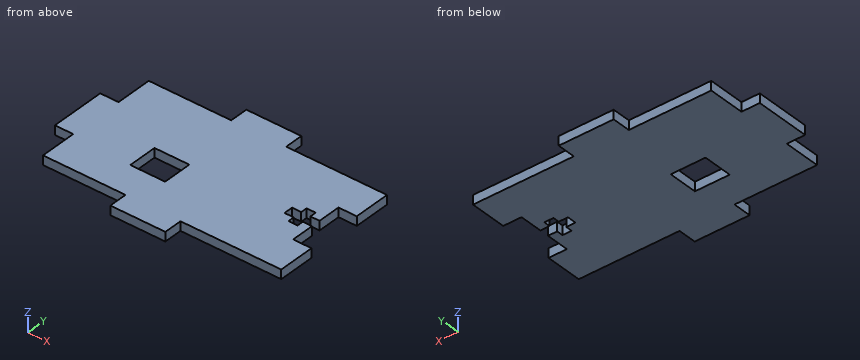
```python
from build123d import *

# Parameters (mm, degrees)
SKETCH1_W           = 82.55
SKETCH1_H           = 44.45
BOSS_EXTRUDE1_DEPTH = 3.175
SKETCH2_W           = 6.35
SKETCH2_H           = 19.05
BOSS_EXTRUDE2_DEPTH = 3.175
SKETCH5_W           = 19.05
SKETCH5_H           = 6.35
BOSS_EXTRUDE3_DEPTH = 3.175
SKETCH3_W           = 6.35
SKETCH3_H           = 19.05
CUT_EXTRUDE1_DEPTH  = 3.175
SKETCH6_W           = 12.065
SKETCH6_H           = 10.16
CUT_EXTRUDE2_DEPTH  = 97.980529618
CUT_EXTRUDE3_DEPTH  = 97.980529618


with BuildPart() as part:
    # Sketch1 → Boss-Extrude1 (new body)
    with BuildSketch(Plane.XY):
        with Locations((41.275, 22.225)):
            Rectangle(SKETCH1_W, SKETCH1_H)
    extrude(amount=BOSS_EXTRUDE1_DEPTH)

    # Sketch2 → Boss-Extrude2 (add)
    with BuildSketch(Plane.XY.offset(3.175)):
        with Locations((-3.175, 22.225)):
            Rectangle(SKETCH2_W, SKETCH2_H)
    extrude(amount=-BOSS_EXTRUDE2_DEPTH)

    # Sketch5 → Boss-Extrude3 (add)
    with BuildSketch(Plane.XY.offset(3.175)):
        with Locations((38.1, 47.625)):
            Rectangle(SKETCH5_W, SKETCH5_H)
        with Locations((38.1, -3.175)):
            Rectangle(SKETCH5_W, SKETCH5_H)
    extrude(amount=-BOSS_EXTRUDE3_DEPTH)

    # Sketch3 → Cut-Extrude1 (cut)
    with BuildSketch(Plane.XY.offset(3.175)):
        with Locations((79.375, 22.225)):
            Rectangle(SKETCH3_W, SKETCH3_H)
    extrude(amount=-CUT_EXTRUDE1_DEPTH, mode=Mode.SUBTRACT)

    # Sketch6 → Cut-Extrude2 (cut, through all)
    with BuildSketch(Plane.XY.offset(3.175)):
        with Locations((26.8605, 16.51)):
            Rectangle(SKETCH6_W, SKETCH6_H)
    extrude(amount=-CUT_EXTRUDE2_DEPTH, mode=Mode.SUBTRACT)

    # Sketch7 → Cut-Extrude3 (cut, through all)
    with BuildSketch(Plane.XY.offset(3.175)):
        Polygon((69.85, 26.035), (73.025, 26.035), (73.025, 23.8125), (76.2, 23.8125), (76.2, 20.6375), (73.025, 20.6375), (73.025, 18.415), (69.85, 18.415), (69.85, 20.6375), (66.675, 20.6375), (66.675, 23.8125), (69.85, 23.8125), align=None)
    extrude(amount=-CUT_EXTRUDE3_DEPTH, mode=Mode.SUBTRACT)


solid = part.part
```
Check sheet for the modelled part. Datum: model origin and axes. Units: mm. Round coordinates to 2 decimals unless told otherwise and drop trailing zeros. Order: outer loops, then holes, each group sorted by start corner. A loop starts at its lowest first (then second) coordinate and runs counter-clockwise, first axis right, second up. Notation, with made-up numbers: M 78.5,-6 L 125.5,-6 A14 cw 125.5,11 Z; hole C 22.25,-0.5 d7. An arc over 180 degrees is marked long. Answer in a Markdown table with one row per item.
(1) Gauge pin test, flat ends, axial feed: pin 1 (1 mm diameter, centred on x = 78, z = 1, fed in from +Y); pin 2 (1 mm diameter, centred on y = 35.5, z = 1, fed in from -X); pin 3 (1 mm diameter, centred on x = 21, y = 18, fed in from +Z) (3 decimals); pin 4 (1.6 mm diameter, centred on x = 74, z = 1, fed in from -Y). Record the tip position at first contact, or that the pin passes through.
Findings:
| item | result |
|---|---|
| pin 1 | stops at y = 44.45 |
| pin 2 | stops at x = 0 |
| pin 3 | stops at z = 3.175 |
| pin 4 | stops at y = 0 |
(2) Material ranges on line 1 along X through (y, z) = (19, 2.2) (3 decimals); line 2 along Y through (x, z) = (74.5, 0.9); line 3 along Y through (x, z) = (27, 0.4), recorded low to high. Write a range as from..to.
Findings:
| item | result |
|---|---|
| line 1 | x = -6.35..20.828, 32.893..69.85, 73.025..76.2 |
| line 2 | y = 0..20.64, 23.81..44.45 |
| line 3 | y = 0..11.43, 21.59..44.45 |
(3) Section check C-C on y = 29.5. Record the boundary of the cut face in (x, z) (3 decimals).
Findings:
| item | result |
|---|---|
| outline | M -6.35,0 L 76.2,0 L 76.2,3.175 L -6.35,3.175 Z |
(4) Section check A-A on x = 24.5. Record the boundary of the cut face in (y, z) (3 decimals), plus the area to 3 significant figures.
Findings:
| item | result |
|---|---|
| outline | M 0,0 L 11.43,0 L 11.43,3.175 L 0,3.175 Z; M 21.59,0 L 44.45,0 L 44.45,3.175 L 21.59,3.175 Z |
| area | 109 mm^2 |
(5) Section check B-B on y = 19.5. Record the boundary of the cut face in (x, z) (3 decimals), plus the area to 3 significant figures.
Findings:
| item | result |
|---|---|
| outline | M -6.35,0 L 20.828,0 L 20.828,3.175 L -6.35,3.175 Z; M 32.893,0 L 69.85,0 L 69.85,3.175 L 32.893,3.175 Z; M 73.025,0 L 76.2,0 L 76.2,3.175 L 73.025,3.175 Z |
| area | 214 mm^2 |
